```python
from build123d import *

# Parameters (mm, degrees)
SKETCH007_R      = 1.05
EXTRUDE008_DEPTH = 30
SKETCH003_R      = 21
SKETCH003_R_2    = 17
EXTRUDE003_DEPTH = 5


with BuildPart() as extrude008:
    # Sketch007 → Extrude008 (new body)
    with BuildSketch(Plane(origin=(-30.396078, 0, 0), x_dir=(0, -1, 0), z_dir=(-1, 0, 0))):
        with Locations((0, 27.512153)):
            Circle(SKETCH007_R)
    extrude(amount=-EXTRUDE008_DEPTH)


with BuildPart() as cut002:
    # Sketch003 (on Face321 of involutegear) → Extrude003 (new body)
    with BuildSketch(Plane(origin=(0, 0, 30), x_dir=(1, 0, 0), z_dir=(0, 0, -1))):
        Circle(SKETCH003_R)
        Circle(SKETCH003_R_2, mode=Mode.SUBTRACT)
    extrude(amount=EXTRUDE003_DEPTH)

    # Cut002: cut Extrude008
    add(extrude008.part, mode=Mode.SUBTRACT)


solid = cut002.part
```
Geometry check sheet. Reference: the model listing, model coordinates, mm. A direction names the side the tool comes from. Round coordinates to 2 decimals unless told otherwise and drop trailing zeros. Loops run counter-clockwise (first coordinate to the right, second up) from the corner with the lowest first, then second, coordinate; pieces in that order, holes last. Notation, with made-up numbers: (-15.5, 10) - (6.5, 10) arc R17 ccw to (6.5, 43) - close; hole circle Ø1 at (-31, -4.5). An arc over 180 degrees is marked (long way). Use a Markdown table: item, result.
Q1. Access from +Z, -Z, +X, -X, +Y, -Y to the whole of each face (thin tool, end or side, straight path). Record for faces 1 (the cylindrical face through (-19.012, 0.137, 28.553)), 2 (the flat face through (7.7, 15.5, 25)).
Solutions:
| item | result |
|---|---|
| face 1 | -X |
| face 2 | -Z, +X, -X, +Y, -Y |
Q2. Cross-section at B-B on x = 0. Record the cut outline in (y, z), plus the area to 3 significant figures.
Solutions:
| item | result |
|---|---|
| outline | (-21, 25) - (-17, 25) - (-17, 30) - (-21, 30) - close; (17, 25) - (21, 25) - (21, 30) - (17, 30) - close |
| area | 40.0 mm2 |
Q3. Go/stop test with flat-tipped pins: P1, Ø3, axis at y = 14, z = 28.5, coming from the +X side; P2, Ø2, axis at y = -12.5, z = 27, coming from the -X side. Record where each tip stops, or that it passes through.
Solutions:
| item | result |
|---|---|
| P1 | stops at x = 16.87 |
| P2 | stops at x = -17.57 |
Q4. Material ranges on line 1 (X direction, y = 0, z = 28.85); line 2 (X direction, y = 0.5, z = 28), recorded low to high.
Solutions:
| item | result |
|---|---|
| line 1 | x = -21 to -17, 17 to 21 |
| line 2 | x = 16.99 to 20.99 |
Q5. Cross-section at A-A on y = 0. Record the cut outline in (x, z), plus the area to 3 significant figures.
Solutions:
| item | result |
|---|---|
| outline | (-21, 25) - (-17, 25) - (-17, 26.46) - (-21, 26.46) - close; (-21, 28.56) - (-17, 28.56) - (-17, 30) - (-21, 30) - close; (17, 25) - (21, 25) - (21, 30) - (17, 30) - close |
| area | 31.6 mm2 |
Q6. Draft check along X on faces 3 (the cylindrical face through (16.215, -5.106, 27.535)), 4 (the flat face through (7.7, 15.5, 30)), 5 (the cylindrical face through (20.03, -6.31, 27.54)). Enter one of: released by +X, released by -X, zero draft, split by the parting line, or undercut.
Solutions:
| item | result |
|---|---|
| face 3 | undercut |
| face 4 | zero draft |
| face 5 | split by the parting line |
Q7. Cross-section at C-C on y = -7.5. Record the cut outline in (x, z), plus the area to 3 significant figures.
Solutions:
| item | result |
|---|---|
| outline | (-19.62, 25) - (-15.26, 25) - (-15.26, 30) - (-19.62, 30) - close; (15.26, 25) - (19.62, 25) - (19.62, 30) - (15.26, 30) - close |
| area | 43.6 mm2 |
